```python
from build123d import *

# Parameters (mm, degrees)
SKETCH_1_R          = 3
EXTRUDE_1_DEPTH     = 0.5
SKETCH_2_R          = 1.5
EXTRUDE_2_DEPTH     = 8
CHAMFER_1_SIZE      = 0.2
CUT_EXTRUDE_1_DEPTH = 0.8
FILLET_2_R          = 0.3


with BuildPart() as part:
    # 草图1 → 凸台-拉伸1 (new body, symmetric)
    with BuildSketch(Plane.XY):
        Circle(SKETCH_1_R)
    extrude(amount=EXTRUDE_1_DEPTH, both=True)

    # 草图2 → 凸台-拉伸2 (add)
    with BuildSketch(Plane(origin=(0, 0, -0.5), x_dir=(-1, 0, 0), z_dir=(0, 0, -1))):
        Circle(SKETCH_2_R)
    extrude(amount=EXTRUDE_2_DEPTH)

    # 倒角1
    chamfer_1_edges = [part.edges().sort_by_distance(p)[0] for p in [
        (1.5, 0, -8.5),
    ]]
    chamfer(chamfer_1_edges, length=CHAMFER_1_SIZE)

    # 草图3 → 切除-拉伸1 (cut)
    with BuildSketch(Plane.XY.offset(0.5)):
        Polygon((1.154700538, 0), (0.577350269, 1), (-0.577350269, 1), (-1.154700538, 0), (-0.577350269, -1), (0.577350269, -1), align=None)
    extrude(amount=-CUT_EXTRUDE_1_DEPTH, mode=Mode.SUBTRACT)

    # 圆角2
    fillet_2_edges = [part.edges().sort_by_distance(p)[0] for p in [
        (-3, 0, -0.5),
        (-3, 0, 0.5),
    ]]
    fillet(fillet_2_edges, radius=FILLET_2_R)


solid = part.part
```
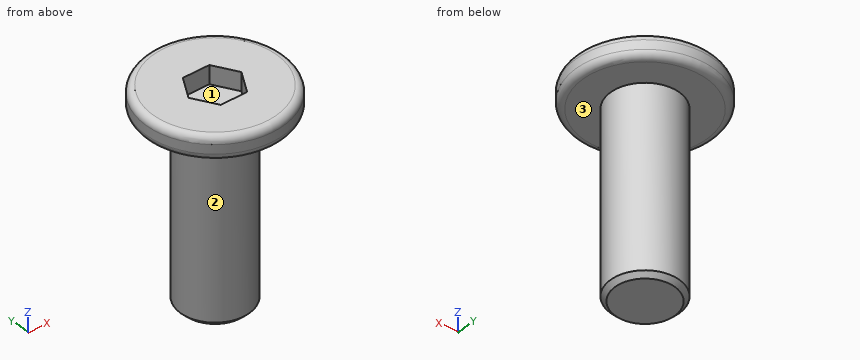
Input: part model. Units: mm. Frame: model coordinates. Face numbers are marked on the shaded views. Coordinates: 2 decimals unless noted, no trailing zeros. Loops run counter-clockwise (first coordinate to the right, second up) from the corner with the lowest first, then second, coordinate; pieces in that order, holes last. Notation, with made-up numbers: M 7,-24.5 L 50,-24.5 A8 ccw 50,-19.5 Z; hole C 60,72 d4. An arc over 180 degrees is marked long. Use a Markdown table: item, result. Add a question column.
1) Pin query (flat end, axial travel): P1, Ø1, axis at x = 0, y = 0, coming from the +Z side; P2, Ø2, axis at x = 1.5, z = -5, coming from the -Y side. Return the tip coordinate at first contact, or that it passes through.
2) Draft query along Y for the marked faces 1, 2 and 3. Return one class per face: +Y half, -Y half, draft (parallel to the pull), parting line (faces both ways), or undercut.
3) Section A-A, the plane x = 0. Return the cut outline in (y, z), plus the area to 3 significant figures.
4) Line query: L1, parallel to Y at x = 0, z = 0; L2, parallel to Z at x = -1, y = 1.5; L3, parallel to Z at x = 0.25, y = 0. Output: solid intervals per line, ascending. Write a range as from..to.
5) Section B-B, the plane z = -1.25. Return the cut outline in (x, y), plus the area to 3 significant figures.
Answer below:
| question | item | result |
|---|---|---|
| 1 | P1 | z = -0.3 |
| 1 | P2 | y = -1.41 |
| 2 | face 1 | undercut |
| 2 | face 2 | parting line |
| 2 | face 3 | draft |
| 3 | outline | M -3,-0.2 A0.3 ccw -2.7,-0.5 L -1.5,-0.5 L -1.5,-8.3 L -1.3,-8.5 L 1.3,-8.5 L 1.5,-8.3 L 1.5,-0.5 L 2.7,-0.5 A0.3 ccw 3,-0.2 L 3,0.2 A0.3 ccw 2.7,0.5 L 1,0.5 L 1,-0.3 L -1,-0.3 L -1,0.5 L -2.7,0.5 A0.3 ccw -3,0.2 Z |
| 3 | area | 28.3 mm2 |
| 4 | L1 | -3..-1, 1..3 |
| 4 | L2 | -0.5..0.5 |
| 4 | L3 | -8.5..-0.3 |
| 5 | outline | C 0,0 d3 |
| 5 | area | 7.07 mm2 |
